from build123d import *

# Parameters (mm, degrees)
SKETCH1_W           = 58
SKETCH1_H           = 65
SKETCH1_R           = 2.5
BOSS_EXTRUDE1_DEPTH = 3.5
SKETCH2_R           = 14.1
SKETCH2_R_2         = 9.75
BOSS_EXTRUDE2_DEPTH = 2.5
SKETCH2_3_R         = 14.1
BOSS_EXTRUDE3_DEPTH = 11
BOSS_EXTRUDE4_START = -54
SKETCH2_4_R         = 14.1
BOSS_EXTRUDE4_DEPTH = 11
BOSS_EXTRUDE5_START = -62.5
SKETCH2_5_R         = 14.1
SKETCH2_5_R_2       = 9.75
BOSS_EXTRUDE5_DEPTH = 2.5
FILLET3_R           = 4
BOSS_EXTRUDE6_REACH = 73.908


with BuildPart() as part:
    # Sketch1 → Boss-Extrude1 (new body)
    with BuildSketch(Plane(origin=(0, 0, 0), x_dir=(1, 0, 0), z_dir=(0, 1, 0))):
        Rectangle(SKETCH1_W, SKETCH1_H)
        with Locations(Location((-25, -16.25, 0), (0, 0, 270))):
            Circle(SKETCH1_R, mode=Mode.SUBTRACT)
        with Locations(Location((25, -16.25, 0), (0, 0, 270))):
            Circle(SKETCH1_R, mode=Mode.SUBTRACT)
        with Locations(Location((25, 16.25, 0), (0, 0, 270))):
            Circle(SKETCH1_R, mode=Mode.SUBTRACT)
        with Locations(Location((-25, 16.25, 0), (0, 0, 270))):
            Circle(SKETCH1_R, mode=Mode.SUBTRACT)
    extrude(amount=BOSS_EXTRUDE1_DEPTH)

    # Sketch2 → Boss-Extrude2 (add)
    # profile 1 of 2: a face of its own
    with BuildSketch(Plane.XY.offset(32.5)):
        with BuildLine():
            ThreePointArc((18.1, 19.5), (0, 37.6), (-18.1, 19.5))
            Line((-18.1, 19.5), (-18.1, 3.5))
            Line((-18.1, 3.5), (18.1, 3.5))
            Line((18.1, 3.5), (18.1, 19.5))
        make_face()
        with Locations((0, 19.5)):
            Circle(SKETCH2_R, mode=Mode.SUBTRACT)
    # profile 2 of 2: a face of its own
    with BuildSketch(Plane.XY.offset(32.5)):
        with Locations((0, 19.5)):
            Circle(SKETCH2_R)
        with Locations((0, 19.5)):
            Circle(SKETCH2_R_2, mode=Mode.SUBTRACT)
    extrude(amount=-BOSS_EXTRUDE2_DEPTH)

    # Sketch2<3> → Boss-Extrude3 (add)
    with BuildSketch(Plane.XY.offset(32.5)):
        with BuildLine():
            ThreePointArc((18.1, 19.5), (0, 37.6), (-18.1, 19.5))
            Line((-18.1, 19.5), (-18.1, 3.5))
            Line((-18.1, 3.5), (18.1, 3.5))
            Line((18.1, 3.5), (18.1, 19.5))
        make_face()
        with Locations((0, 19.5)):
            Circle(SKETCH2_3_R, mode=Mode.SUBTRACT)
    extrude(amount=-BOSS_EXTRUDE3_DEPTH)

    # Sketch2<4> → Boss-Extrude4 (add)
    with BuildSketch(Plane.XY.offset(32.5).offset(BOSS_EXTRUDE4_START)):
        with BuildLine():
            ThreePointArc((18.1, 19.5), (0, 37.6), (-18.1, 19.5))
            Line((-18.1, 19.5), (-18.1, 3.5))
            Line((-18.1, 3.5), (-29, 3.5))
            Line((-29, 3.5), (-29, 0))
            Line((-29, 0), (29, 0))
            Line((29, 0), (29, 3.5))
            Line((29, 3.5), (18.1, 3.5))
            Line((18.1, 3.5), (18.1, 19.5))
        make_face()
        with Locations((0, 19.5)):
            Circle(SKETCH2_4_R, mode=Mode.SUBTRACT)
    extrude(amount=-BOSS_EXTRUDE4_DEPTH)

    # Sketch2<5> → Boss-Extrude5 (add)
    with BuildSketch(Plane.XY.offset(32.5).offset(BOSS_EXTRUDE5_START)):
        with Locations((0, 19.5)):
            Circle(SKETCH2_5_R)
        with Locations((0, 19.5)):
            Circle(SKETCH2_5_R_2, mode=Mode.SUBTRACT)
    extrude(amount=-BOSS_EXTRUDE5_DEPTH)

    # Fillet3
    fillet3_edges = [part.edges().sort_by_distance(p)[0] for p in [
        (18.1, 3.5, 27),
        (-18.1, 3.5, 27),
        (-18.1, 3.5, -27),
        (18.1, 3.5, -27),
    ]]
    fillet(fillet3_edges, radius=FILLET3_R)

    # Sketch6 → Boss-Extrude6 (add, up to next)
    with BuildSketch(Plane.XY.offset(-21.5), mode=Mode.PRIVATE) as boss_extrude6_sk1:
        with BuildLine():
            Line((-18.1, 7.5), (-18.1, 19.5))
            Line((-18.1, 19.5), (-14.1, 19.5))
            ThreePointArc((-14.1, 19.5), (0, 5.4), (14.1, 19.5))
            Line((14.1, 19.5), (18.1, 19.5))
            Line((18.1, 19.5), (18.1, 7.5))
            ThreePointArc((18.1, 7.5), (19.271572875, 4.671572875), (22.1, 3.5))
            Line((22.1, 3.5), (-22.1, 3.5))
            ThreePointArc((-22.1, 3.5), (-19.271572875, 4.671572875), (-18.1, 7.5))
        make_face()
    boss_extrude6_tool1 = extrude(boss_extrude6_sk1.sketch, amount=BOSS_EXTRUDE6_REACH, mode=Mode.PRIVATE) - part.part
    add(boss_extrude6_tool1.solids().sort_by_distance((-18.939185, 4.339185, -21.5))[0])


solid = part.part
Could you check a few things on this model? Use its own coordinates, in mm. A direction names the side the tool comes from. Give positions to 0.01 mm unless a question says otherwise; leave off trailing zeros. Order: outer loops, then holes, each group sorted by start corner. A loop starts at its lowest first (then second) coordinate and runs counter-clockwise, first axis right, second up.
1. We'd pull the mould along Z, two halves only. Please class faces 6 (the flat face through (-7, 11, 32.5)), 7 (the flat face through (-18.1, 13, 0)), 8 (the flat face through (-16, 19.5, 0)): pulls with the +Z half, pulls with the -Z half, needs draft (parallel to the pull), parting line crosses it, or undercut.
2. Suppose I cut it at A-A (x = 25). List the corners of the cut face in (y, z) for me.
3. For faces 1 (the flat face through (-3, 10, -30)), 2 (the cylindrical face through (0.398, 37.596, 27.077)), 3 (the flat face through (1, 34, 21.5)), 4 (the cylindrical face through (-23.31, 1.73, -18.09)), 5 (the flat face through (26, 3.5, 0)), which set-ups out of +Z, -Z, +X, -X, +Y, -Y let a thin tool reach every point of the face, with its end or its side?
4. Suppose I cut it at C-C (z = 27). List the corners of the cut face in (x, y) for me.
5. Suppose I cut it at B-B (z = -16.25). List the corners of the cut face in (x, y) for me, plus the area to 3 significant figures.
6. Will these pins go through, and if not, where does the flat tip stop? P1, Ø3.5, axis at x = -26, z = 5.5, coming from the +Y side; P2, Ø10, axis at y = 11, z = -8.5, coming from the -X side; P3, Ø1.2, axis at x = 16, z = -3, coming from the +Y side; P4, Ø20, axis at x = -0.5, y = 28.5, coming from the -Z side.
7. I need wall thicknesses on L1, parallel to X at y = 1.65, z = 16.25; L2, parallel to Z at x = -8.5, y = 11.5; L3, parallel to Y at x = 0, z = 31.8. Which ranges of each line are inside material? Lowest first, please.
8. Suppose I cut it at D-D (x = 0). List the corners of the cut face in (y, z) for me, plus the area to 4 significant figures.
Solved:
1. face 6: pulls with the +Z half
1. face 7: needs draft
1. face 8: undercut
2. outline: (0, -32.5) - (3.5, -32.5) - (3.5, -18.75) - (0, -18.75) - close; (0, -13.75) - (3.5, -13.75) - (3.5, 13.75) - (0, 13.75) - close; (0, 18.75) - (3.5, 18.75) - (3.5, 32.5) - (0, 32.5) - close
3. face 1: none
3. face 2: +Z, -Z, +Y
3. face 3: +X, -X, +Y
3. face 4: +Y, -Y
3. face 5: +Z, -Z, +X, +Y
4. outline: (-29, 0) - (29, 0) - (29, 3.5) - (22.1, 3.5) arc R4 cw to (18.1, 7.5) - (18.1, 19.5) arc R18.1 ccw to (-18.1, 19.5) - (-18.1, 7.5) arc R4 cw to (-22.1, 3.5) - (-29, 3.5) - close; hole circle Ø28.2 at (0, 19.5)
5. outline: (-29, 0) - (-27.5, 0) - (-27.5, 3.5) - (-29, 3.5) - close; (-22.5, 0) - (22.5, 0) - (22.5, 3.5) - (22.1, 3.5) arc R4 cw to (18.1, 7.5) - (18.1, 19.5) - (14.1, 19.5) arc R14.1 cw to (-14.1, 19.5) - (-18.1, 19.5) - (-18.1, 7.5) arc R4 cw to (-22.1, 3.5) - (-22.5, 3.5) - close; (27.5, 0) - (29, 0) - (29, 3.5) - (27.5, 3.5) - close
5. area: 442 mm2
6. P1: stops at y = 3.5
6. P2: stops at x = -18.39
6. P3: stops at y = 19.5
6. P4: stops at z = -32.5
7. L1: x = -29 to -27.5, -22.5 to 22.5, 27.5 to 29
7. L2: z = -32.5 to -30, 30 to 32.5
7. L3: y = 0 to 9.75, 29.25 to 37.6
8. outline: (0, -32.5) - (9.75, -32.5) - (9.75, -30) - (5.4, -30) - (5.4, 30) - (9.75, 30) - (9.75, 32.5) - (0, 32.5) - close; (29.25, -32.5) - (37.6, -32.5) - (37.6, -21.5) - (33.6, -21.5) - (33.6, -30) - (29.25, -30) - close; (29.25, 30) - (33.6, 30) - (33.6, 21.5) - (37.6, 21.5) - (37.6, 32.5) - (29.25, 32.5) - close
8. area: 482.5 mm2
